The listing builds one solid part. Answer for the finished solid, in the listing's coordinates (mm). A direction names the side the tool comes from. Coordinates: 2 decimals unless noted, no trailing zeros. Write each loop counter-clockwise with the first axis right and the second up, starting at its lowest first coordinate (ties: lowest second). Pieces come first, ordered by that corner, then holes. Notation, with made-up numbers: M 5,10 L 24,10 A13 cw 24,26 Z; hole C 9,30.25 d8. An arc over 180 degrees is marked long. Answer as CSV lines item,"result".
```python
from build123d import *

# Parameters (mm, degrees)
EXTRUDE_1_DEPTH      = 6
SKETCH_2_W           = 7
SKETCH_2_H           = 6
EXTRUDE_2_DEPTH      = 6
CUT_EXTRUDE_1_DEPTH  = 7
SKETCH_21_W          = 7
SKETCH_21_H          = 6
EXTRUDE_21_DEPTH     = 6
SKETCH_22_W          = 7
SKETCH_22_H          = 6
EXTRUDE_22_DEPTH     = 6
CUT_EXTRUDE_12_DEPTH = 7
SKETCH_23_W          = 7
SKETCH_23_H          = 6
EXTRUDE_24_DEPTH     = 6


with BuildPart() as part:
    # Эскиз1 → Бобышка-Вытянуть1 (new body)
    with BuildSketch(Plane.XY):
        with BuildLine():
            Line((-44.810940225, 6.078379342), (-3.810940225, 6.078379342))
            Line((-3.810940225, 6.078379342), (-1.488167872, 6.078379342))
            Line((-1.488167872, 6.078379342), (-1.488167872, 8.8692773))
            ThreePointArc((-1.488167872, 8.8692773), (-1.754354552, 10.10469817), (-2.50567769, 11.120883988))
            Line((-2.50567769, 11.120883988), (-35.394057565, 40.078379342))
            Line((-35.394057565, 40.078379342), (-44.810940225, 40.078379342))
            Line((-44.810940225, 40.078379342), (-44.810940225, 6.078379342))
        make_face()
    extrude(amount=-EXTRUDE_1_DEPTH)

    # Эскиз2 → Бобышка-Вытянуть2 (add)
    with BuildSketch(Plane(origin=(5.189059775, 23.078379342, -6), x_dir=(0, -1, 0), z_dir=(0, 0, -1))):
        with Locations((-9.531849908, 53)):
            Rectangle(SKETCH_2_W, SKETCH_2_H)
        with Locations((9.531849908, 53)):
            Rectangle(SKETCH_2_W, SKETCH_2_H)
    extrude(amount=-EXTRUDE_2_DEPTH)

    # Эскиз3 → Вырез-Вытянуть1 (cut, through all)
    with BuildSketch(Plane(origin=(5.189059775, 23.078379342, -6), x_dir=(0, -1, 0), z_dir=(0, 0, -1))):
        Polygon((-2.1, 45), (-3.6, 45), (-3.6, 42.6), (-2.1, 42.6), (-2.1, 39), (2.1, 39), (2.1, 42.6), (3.6, 42.6), (3.6, 45), (2.1, 45), (2.1, 50), (-2.1, 50), align=None)
    extrude(amount=-CUT_EXTRUDE_1_DEPTH, mode=Mode.SUBTRACT)

    # Эскиз21 → Бобышка-Вытянуть21 (add)
    with BuildSketch(Plane(origin=(5.189059775, 23.078379342, 0), x_dir=(0, 1, 0), z_dir=(0, 0, 1))):
        with Locations((-9.531849908, 53)):
            Rectangle(SKETCH_21_W, SKETCH_21_H)
        with Locations((9.531849908, 53)):
            Rectangle(SKETCH_21_W, SKETCH_21_H)
    extrude(amount=-EXTRUDE_21_DEPTH)

    # Эскиз22 → Бобышка-Вытянуть22 (add)
    with BuildSketch(Plane(origin=(-21.488167872, 56.078379342, 0), x_dir=(-1, 0, 0), z_dir=(0, 0, 1))):
        with Locations((-9.531849908, 53)):
            Rectangle(SKETCH_22_W, SKETCH_22_H)
        with Locations((9.531849908, 53)):
            Rectangle(SKETCH_22_W, SKETCH_22_H)
    extrude(amount=-EXTRUDE_22_DEPTH)

    # Эскиз32 → Вырез-Вытянуть12 (cut, through all)
    with BuildSketch(Plane(origin=(-21.488167872, 56.078379342, 0), x_dir=(-1, 0, 0), z_dir=(0, 0, 1))):
        Polygon((-2.1, 45), (-3.6, 45), (-3.6, 42.6), (-2.1, 42.6), (-2.1, 37.5), (2.1, 37.5), (2.1, 42.6), (3.6, 42.6), (3.6, 45), (2.1, 45), (2.1, 50), (-2.1, 50), align=None)
    extrude(amount=-CUT_EXTRUDE_12_DEPTH, mode=Mode.SUBTRACT)

    # Эскиз23 → Бобышка-Вытянуть24 (add)
    with BuildSketch(Plane(origin=(-21.488167872, 56.078379342, -6), x_dir=(1, 0, 0), z_dir=(0, 0, -1))):
        with Locations((-9.531849908, 53)):
            Rectangle(SKETCH_23_W, SKETCH_23_H)
        with Locations((9.531849908, 53)):
            Rectangle(SKETCH_23_W, SKETCH_23_H)
    extrude(amount=-EXTRUDE_24_DEPTH)


solid = part.part
```
Q1. For faces 5 (the flat face through (-39.811, 20, -3)), 6 (the flat face through (-27.52, 3, -3)), 7 (the flat face through (-8.456, 3, -3)), determine the directions among +Z, -Z, +X, -X, +Y, -Y from which every point of the face is accessible in a straight line to the end or side of a thin tool.
Output:
face 5,"+Z, -Z"
face 6,"+Z, -Z, -Y"
face 7,"+Z, -Z, +X, -Y"
Q2. Find section B-B (y = 14). Give the vertices of the cut face in (x, z), and give its area (3 significant figures).
Output:
outline,"M -50.81,-6 L -23.59,-6 L -23.59,0 L -50.81,0 Z; M -19.39,-6 L -5.78,-6 L -5.78,0 L -19.39,0 Z"
area,"245 mm2"
Q3. Flat-ended cylindrical pins translate along their axes: pin 1 Ø2 at (y, z) = (19.5, -4) entering from -X; pin 2 Ø3 at (x, z) = (-46.5, -4.5) entering from +Y; pin 3 Ø1.2 at (y, z) = (26, -2.5) entering from +X. Find the tip coordinate at first contact, or state that the pin passes through.
Output:
pin 1,"x = -44.81"
pin 2,"y = 36.11"
pin 3,"x = -18.72"
Q4. Find section C-C (x = -6). Give the vertices of the cut face in (y, z).
Output:
outline,"M 6.08,-6 L 14.2,-6 L 14.2,0 L 6.08,0 Z"
Q5. Find section A-A (x = -42). Give the vertices of the cut face in (y, z), and give its area (3 significant figures).
Output:
outline,"M 6.08,-6 L 20.98,-6 L 20.98,0 L 6.08,0 Z; M 25.18,-6 L 40.08,-6 L 40.08,0 L 25.18,0 Z"
area,"179 mm2"
Q6. The mould has two halves that part along Y. Classify faces 1 (the flat face through (-50.811, 33, -3)), 2 (the flat face through (-21, 18.578, -3)), 3 (the flat face through (-37.411, 20, -3)), 4 (the flat face through (-33.811, 23, -3)): pulls with the +Y half, pulls with the -Y half, needs draft (parallel to the pull), parting line crosses it, or undercut.
Output:
face 1,"needs draft"
face 2,"pulls with the -Y half"
face 3,"undercut"
face 4,"undercut"
Q7. Find section D-D (y = 37). Give the vertices of the cut face in (x, z), and give its area (3 significant figures).
Output:
outline,"M -44.81,-6 L -31.9,-6 L -31.9,0 L -44.81,0 Z"
area,"77.5 mm2"
Q8. Straight lines are drawn through the part: line 1 (Y direction, x = -39, z = -1.15); line 2 (X direction, y = 5.5, z = -4.5); line 3 (Y direction, x = -40, z = -4.6). For each, find the intervals that lie inside material, in ascending order.
Output:
line 1,"6.08 to 19.48, 26.68 to 40.08"
line 2,"-34.52 to -27.52, -15.46 to -8.46"
line 3,"6.08 to 20.98, 25.18 to 40.08"
